The model under review builds one solid part; all positions refer to its coordinate system, in mm. Coordinates: 2 decimals unless noted, no trailing zeros. Write each loop counter-clockwise with the first axis right and the second up, starting at its lowest first coordinate (ties: lowest second). Pieces come first, ordered by that corner, then holes. Notation, with made-up numbers: (-25, 33.5) - (16, 33.5) arc R14 ccw to (16, 39.5) - close; hole circle Ø1 at (-29.5, 41). An arc over 180 degrees is marked (long way). Return JSON: item names as keys, results as strings. Group by question number.
(1) We need section C-C on x = -14. State the section outline as (y, z) points.
(2) To check wall thickness, follow L1, parallel to X at y = -5, z = 47.5; L2, parallel to Y at x = 17, z = 41.5; L3, parallel to Z at x = -1, y = 11.25. State the ranges of each line that lie inside material, in increasing order. Write a range as from..to.
(3) We need section D-D on z = 14. State the section outline as (x, y) points, then the cut area to 3 significant figures.
(4) For pin 1 Ø12 at (x, z) = (-15, 47.5) entering from +Y; pin 2 Ø6.5 at (x, z) = (12.5, 49) entering from -Y; pin 3 Ø3 at (x, y) = (4.5, 10) entering from -Z; pin 4 Ø2 at (x, y) = (-20, -1.5) entering from -Z, all flat-tipped, find the tip position at first contact; note any pin that passes through.
(5) We need section B-B on y = 2. State the section outline as (x, z) points, then the cut area to 3 significant figures.
(6) We need section A-A on z = 47.5. State the section outline as (x, y) points.
Autodesk Inventor part; units mm, degrees
ref_plane "YZ Plane" through (0, 0, 0) normal (1, 0, 0) x (0, 1, 0)
ref_plane "XZ Plane" through (0, 0, 0) normal (0, 1, 0) x (-1, 0, 0)
ref_plane "XY Plane" through (0, 0, 0) normal (0, 0, 1) x (1, 0, 0)
sketch "Sketch1" plane through (0, 0, 0) normal (0, 1, 0) x (-1, 0, 0)
  line L0 (30, 60) -> (-30, 60)
  line L1 (-30, 60) -> (-30, 0)
  arc A0 (-30, 0) -> (30, 0) centre (0, 0) ccw
  line L2 (30, 0) -> (30, 60)
  circle A1 centre (0, 0) radius 15
  dimension "d0" = 60
  dimension "d1" = 60
  dimension "d2" = 30
extrude "Extrusion1" add sketch "Sketch1" along normal mid plane 25
sketch "Sketch2" plane through (0, 0, 0) normal (0, 1, 0) x (-1, 0, 0)
  line L0 (-30, 0) -> (-30, 60) construction
  line L1 (-30, 60) -> (30, 60) construction
  line L2 (30, 60) -> (30, 0) construction
  arc A0 (-30, 0) -> (30, 0) centre (0, 0) ccw construction
  circle A1 centre (0, 0) radius 15 construction
  line L3 (30, 60) -> (30, 0) construction
  line L4 (30, 35) -> (-30, 35) construction
  circle A2 centre (15, 47.5) radius 4.05
  line L5 (0, 35) -> (0, 60) construction
  circle A3 centre (-15, 47.5) radius 4.05
  point P0 (0, -30)
  point P1 (0, 47.5)
  dimension "d5" = 65
  dimension "d6" = 8.1
  dimension "d7" = 30
extrude "Extrusion2" cut sketch "Sketch2" along normal through all both and the other way through all
sketch "Sketch3" plane through (0, -12.5, 0) normal (0, -1, 0) x (1, 0, 0)
  circle A0 centre (-15, 47.5) radius 4.05 construction
  circle A1 centre (15, 47.5) radius 4.05 construction
  line L0 (30, 0) -> (30, 60) construction
  line L1 (30, 60) -> (-30, 60) construction
  line L2 (-30, 60) -> (-30, 0) construction
  arc A2 (-30, 0) -> (30, 0) centre (0, 0) ccw construction
  circle A3 centre (0, 0) radius 15 construction
  circle A4 centre (-15, 47.5) radius 6.55
  circle A5 centre (15, 47.5) radius 4.05
  circle A6 centre (15, 47.5) radius 6.55
  dimension "d10" = 13.1
  dimension "d11" = 13.1
extrude "Extrusion3" cut sketch "Sketch3" against normal blind 3 contours A4 | A5 | A6
properties part number "element1_obj4"
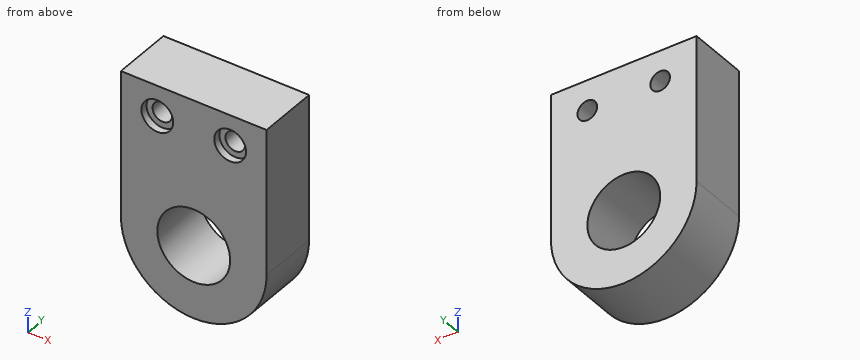
Ans:
{
 "1": {"outline": "(-12.5, -26.53) - (12.5, -26.53) - (12.5, -5.39) - (-12.5, -5.39) - close; (-12.5, 5.39) - (12.5, 5.39) - (12.5, 43.58) - (-9.5, 43.58) - (-9.5, 41.03) - (-12.5, 41.03) - close; (-12.5, 53.97) - (-9.5, 53.97) - (-9.5, 51.42) - (12.5, 51.42) - (12.5, 60) - (-12.5, 60) - close"},
 "2": {"L1": "-30..-19.05, -10.95..10.95, 19.05..30", "L2": "-9.5..12.5", "L3": "-29.98..-14.97, 14.97..60"},
 "3": {"outline": "(-30, -12.5) - (-5.39, -12.5) - (-5.39, 12.5) - (-30, 12.5) - close; (5.39, -12.5) - (30, -12.5) - (30, 12.5) - (5.39, 12.5) - close", "area": "1,230 mm²"},
 "4": {"pin 1": "y = 12.5", "pin 2": "y = -9.5", "pin 3": "z = -29.85", "pin 4": "z = -23.22"},
 "5": {"outline": "(-30, 0) arc R30 ccw to (30, 0) - (30, 60) - (-30, 60) - close; hole circle Ø8.1 at (-15, 47.5); hole circle Ø30 at (0, 0); hole circle Ø8.1 at (15, 47.5)", "area": "4,200 mm²"},
 "6": {"outline": "(-30, -12.5) - (-21.55, -12.5) - (-21.55, -9.5) - (-19.05, -9.5) - (-19.05, 12.5) - (-30, 12.5) - close; (-10.95, -9.5) - (-8.45, -9.5) - (-8.45, -12.5) - (8.45, -12.5) - (8.45, -9.5) - (10.95, -9.5) - (10.95, 12.5) - (-10.95, 12.5) - close; (19.05, -9.5) - (21.55, -9.5) - (21.55, -12.5) - (30, -12.5) - (30, 12.5) - (19.05, 12.5) - close"}
}
